Source: CAD feature listing. Evaluate the final solid. Frame: model axes, mm. Face numbers are marked on the shaded views. Give positions to 0.01 mm unless a question says otherwise; leave off trailing zeros. Loops run counter-clockwise (first coordinate to the right, second up) from the corner with the lowest first, then second, coordinate; pieces in that order, holes last. Notation, with made-up numbers: (-37.75, -6) - (-12.75, -6) arc R20 cw to (-12.75, 2) - close; hole circle Ø9 at (-6, 10). An arc over 180 degrees is marked (long way). Write each question's results on one line, items separated by ' | '. Start each with the question number.
(1) Pull-direction query (X, two-part tool) for the marked faces 1, 2 and 3; classes: pulls with the +X half, pulls with the -X half, needs draft (parallel to the pull), parting line crosses it, or undercut.
(2) Contact query for a flat-ended pin moving along its axis: pin 1 (2 mm diameter, centred on x = 1, y = -0.5, fed in from +Z). Output: stop coordinate, or through.
(3) Material intervals for line 1 along Y through (x, z) = (0, 6.5); line 2 along Z through (x, y) = (-1.1, -1.25); line 3 along Y through (x, z) = (-1.8, 2), sorted ascending. Write a range as [from, to].
(4) Cut plane A-A on y = 0. Return the cut outline in (x, z).
(5) Cut plane B-B on z = 3.25. Return the cut outline in (x, y), then the cut area to 3 significant figures.
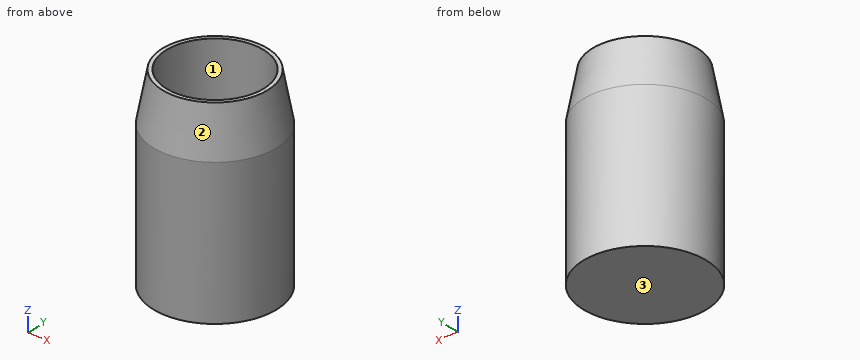
from build123d import *


with BuildPart() as f1:
    # F0 (on Front) → F1 (revolve)
    with BuildSketch(Plane.XZ):
        with BuildLine():
            Line((2.4257, 8.89), (2.2479, 8.89))
            Line((2.2479, 8.89), (2.2479, 1.397))
            ThreePointArc((2.2479, 1.397), (2.210703, 1.307197), (2.1209, 1.27))
            Line((2.1209, 1.27), (0, 1.27))
            Line((0, 1.27), (0, 0))
            Line((0, 0), (2.8448, 0))
            Line((2.8448, 0), (2.8448, 6.662339))
            Line((2.8448, 6.662339), (2.4257, 8.89))
        make_face()
    revolve(axis=Axis((0, 0, 7.564645), (0, 0, 1)))


solid = f1.part
Ans:
1) face 1: undercut | face 2: parting line crosses it | face 3: needs draft
2) pin 1: z = 1.27
3) line 1: [-2.84, -2.25], [2.25, 2.84] | line 2: [0, 1.27] | line 3: [-2.2, -1.35], [1.35, 2.2]
4) outline: (-2.84, 0) - (2.84, 0) - (2.84, 6.66) - (2.43, 8.89) - (2.25, 8.89) - (2.25, 1.4) arc R0.13 cw to (2.12, 1.27) - (-2.12, 1.27) arc R0.13 cw to (-2.25, 1.4) - (-2.25, 8.89) - (-2.43, 8.89) - (-2.84, 6.66) - close
5) outline: circle Ø5.69 at (0, 0); hole circle Ø4.5 at (0, 0) | area: 9.55 mm^2
